Geometry check sheet. Reference: drawing and pictorial views, mm from the part's lowest x, y, z. A direction names the side the tool comes from. Coordinates: 2 decimals unless noted, no trailing zeros. Write each loop counter-clockwise with the first axis right and the second up, starting at its lowest first coordinate (ties: lowest second). Pieces come first, ordered by that corner, then holes. Notation, with made-up numbers: (37.5, 13.5) -> (42.5, 13.5) arc R34 cw to (42.5, 50.5) -> close; hole circle Ø7 at (52, -40). An arc over 180 degrees is marked (long way). Use a Markdown table: item, result.
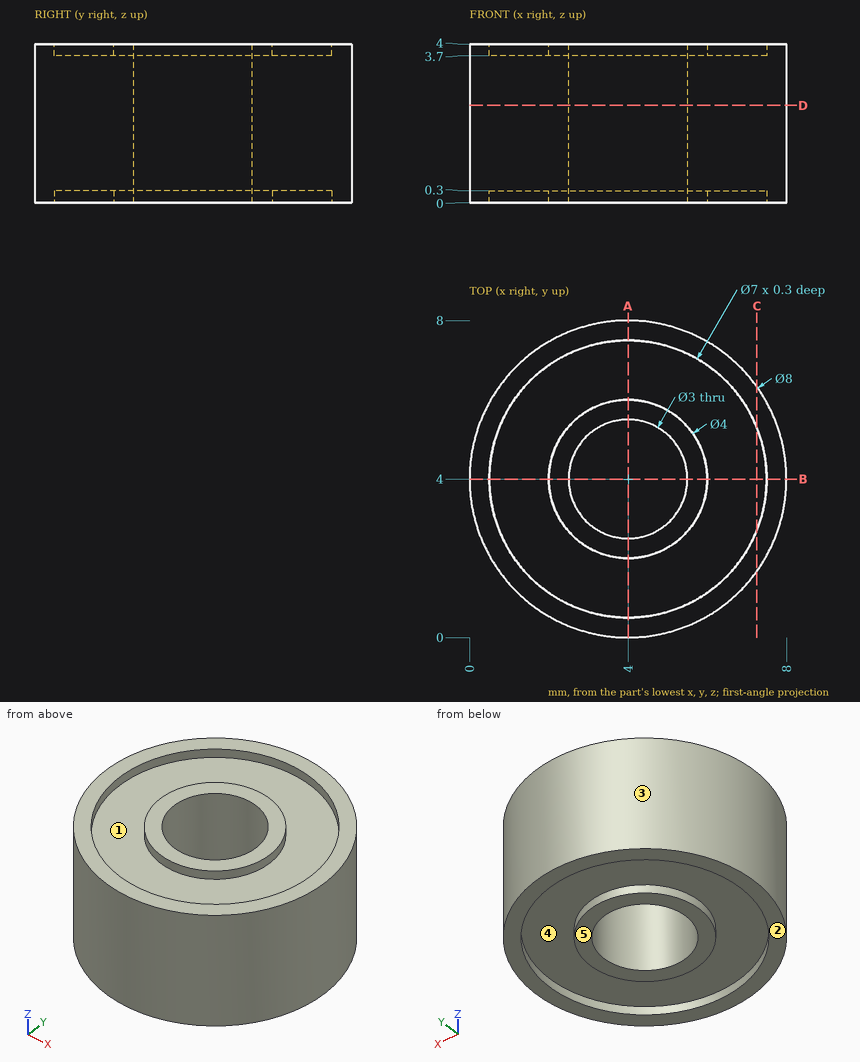
Item 1: Mould release check, pull along X, two halves, no side actions. Record for the marked faces 1, 2 and 3: +X half, -X half, draft (parallel to the pull), parting line (faces both ways), or undercut.
Answer block:
| item | result |
|---|---|
| face 1 | undercut |
| face 2 | draft |
| face 3 | parting line |
Item 2: Section check D-D on z = 2.45. Record the boundary of the cut face in (x, y), then the cut area to 3 significant figures.
Answer block:
| item | result |
|---|---|
| outline | circle Ø8 at (4, 4); hole circle Ø3 at (4, 4) |
| area | 43.2 mm^2 |
Item 3: Tool access check on the marked faces 4 and 5. Record the directions out of +Z, -Z, +X, -X, +Y, -Y that give a thin tool (end or side, any length) a straight path to the whole face; none if there is none.
Answer block:
| item | result |
|---|---|
| face 4 | -Z |
| face 5 | -Z, +X, -X, +Y, -Y |
Item 4: Thickness scan on L1, parallel to Y at x = 4, z = 3.95; L2, parallel to Y at x = 4.25, z = 2.05; L3, parallel to X at y = 3, z = 3. Record the ranges inside material, lowest first. Write a range as [from, to].
Answer block:
| item | result |
|---|---|
| L1 | y = [0, 0.5], [2, 2.5], [5.5, 6], [7.5, 8] |
| L2 | y = [0.01, 2.52], [5.48, 7.99] |
| L3 | x = [0.13, 2.88], [5.12, 7.87] |
Item 5: Section check C-C on x = 7.25. Record the boundary of the cut face in (y, z), then the cut area to 3 significant figures.
Answer block:
| item | result |
|---|---|
| outline | (1.67, 0) -> (2.7, 0) -> (2.7, 0.3) -> (5.3, 0.3) -> (5.3, 0) -> (6.33, 0) -> (6.33, 4) -> (5.3, 4) -> (5.3, 3.7) -> (2.7, 3.7) -> (2.7, 4) -> (1.67, 4) -> close |
| area | 17.1 mm^2 |
Item 6: Depth check by flat-ended pin: P1, Ø1.5, axis at y = 6, z = 1, coming from the -X side. Enter the tip coordinate at first touch or a pass-through.
Answer block:
| item | result |
|---|---|
| P1 | stops at x = 0.2 |
Item 7: Section check A-A on x = 4. Record the boundary of the cut face in (y, z), then the cut area to 3 significant figures.
Answer block:
| item | result |
|---|---|
| outline | (0, 0) -> (0.5, 0) -> (0.5, 0.3) -> (2, 0.3) -> (2, 0) -> (2.5, 0) -> (2.5, 4) -> (2, 4) -> (2, 3.7) -> (0.5, 3.7) -> (0.5, 4) -> (0, 4) -> close; (5.5, 0) -> (6, 0) -> (6, 0.3) -> (7.5, 0.3) -> (7.5, 0) -> (8, 0) -> (8, 4) -> (7.5, 4) -> (7.5, 3.7) -> (6, 3.7) -> (6, 4) -> (5.5, 4) -> close |
| area | 18.2 mm^2 |
